Geometry check sheet. Reference: drawing and pictorial views, mm from the part's lowest x, y, z. A direction names the side the tool comes from. Give positions to 0.01 mm unless a question says otherwise; leave off trailing zeros. Write each loop counter-clockwise with the first axis right and the second up, starting at its lowest first coordinate (ties: lowest second). Pieces come first, ordered by that corner, then holes. Notation, with made-up numbers: (66, 62.5) -> (88, 62.5) arc R10 cw to (88, 66.5) -> close; hole circle Ø11 at (-10.75, -19). An arc over 180 degrees is marked (long way). Use a Markdown table: item, result. Add a question column.
1. Cross-section at D-D (y = 14). Enter the section's corners in (x, z).
2. Cross-section at C-C (x = 8.5). Enter the section's corners in (y, z).
3. Cross-section at B-B (z = 0.8). Enter the section's corners in (x, y), then the cut area to 3 significant figures.
4. Set-up check for the marked faces 1 and 2: record each of +Z, -Z, +X, -X, +Y, -Y from which the full face is reachable in a straight line by a thin tool's end or side.
5. Release check for a two-part mould opening along Y. For the marked faces 3 and 4 record: released by +Y, released by -Y, zero draft, split by the parting line, or undercut.
6. Cross-section at A-A (x = 11.75). Enter the section's corners in (y, z), then the cut area to 3 significant figures.
7. Scan lines: probe 1 along Y at (x, z) = (21, 3.7); probe 2 along X at (y, z) = (50, 0.5) (1 decimal); probe 3 along Z at (x, y) = (2, 4). Record each from-to range of solid material in increasing order. Write a range as [from, to].
8. Gauge pin test, flat ends, axial feed: P1, Ø4, axis at x = 2.14, y = 49.49, coming from the +Z side; P2, Ø1.5, axis at x = 18, z = 1, coming from the -Y side; P3, Ø2, axis at y = 49, z = 1, coming from the -X side; P4, Ø2.5, axis at x = 19.44, y = 49.49, coming from the -Z side. Record the tip position at first contact, or that the pin passes through.
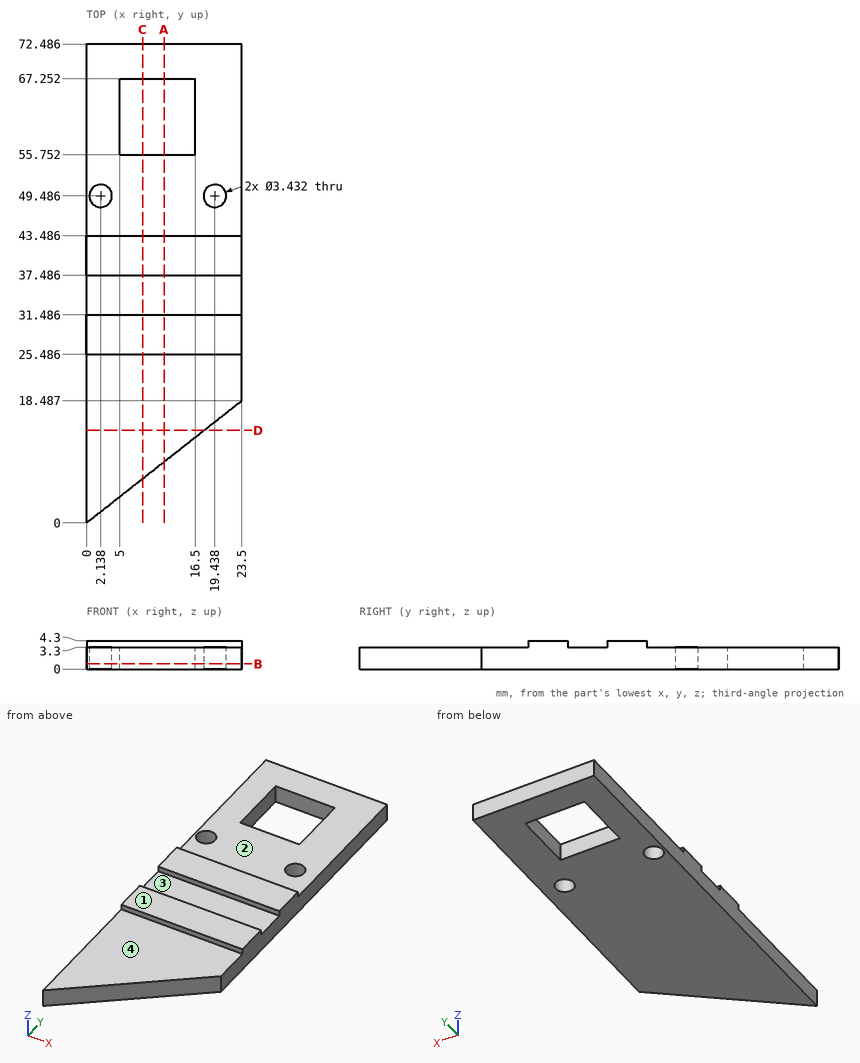
Worked answers:
| question | item | result |
|---|---|---|
| 1 | outline | (0, 0) -> (17.8, 0) -> (17.8, 3.3) -> (0, 3.3) -> close |
| 2 | outline | (6.69, 0) -> (55.75, 0) -> (55.75, 3.3) -> (43.49, 3.3) -> (43.49, 4.3) -> (37.49, 4.3) -> (37.49, 3.3) -> (31.49, 3.3) -> (31.49, 4.3) -> (25.49, 4.3) -> (25.49, 3.3) -> (6.69, 3.3) -> close; (67.25, 0) -> (72.49, 0) -> (72.49, 3.3) -> (67.25, 3.3) -> close |
| 3 | outline | (0, 0) -> (23.5, 18.49) -> (23.5, 72.49) -> (0, 72.49) -> close; hole circle Ø3.43 at (2.14, 49.49); hole (5, 55.75) -> (16.5, 55.75) -> (16.5, 67.25) -> (5, 67.25) -> close; hole circle Ø3.43 at (19.44, 49.49) |
| 3 | area | 1,340 mm² |
| 4 | face 1 | +Z, +X, -X, +Y, -Y |
| 4 | face 2 | +Z, +X, -X, +Y |
| 5 | face 3 | undercut |
| 5 | face 4 | zero draft |
| 6 | outline | (9.24, 0) -> (55.75, 0) -> (55.75, 3.3) -> (43.49, 3.3) -> (43.49, 4.3) -> (37.49, 4.3) -> (37.49, 3.3) -> (31.49, 3.3) -> (31.49, 4.3) -> (25.49, 4.3) -> (25.49, 3.3) -> (9.24, 3.3) -> close; (67.25, 0) -> (72.49, 0) -> (72.49, 3.3) -> (67.25, 3.3) -> close |
| 6 | area | 183 mm² |
| 7 | probe 1 | y = [25.49, 31.49], [37.49, 43.49] |
| 7 | probe 2 | x = [0, 0.5], [3.8, 17.8], [21.1, 23.5] |
| 7 | probe 3 | z = [0, 3.3] |
| 8 | P1 | stops at z = 3.3 |
| 8 | P2 | stops at y = 13.57 |
| 8 | P3 | stops at x = 0 |
| 8 | P4 | passes through |
